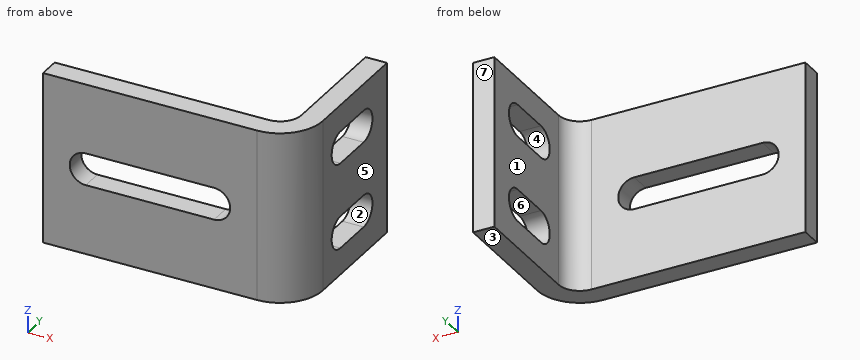
Autodesk Inventor part; units mm, degrees
ref_plane "YZ Plane" through (0, 0, 0) normal (1, 0, 0) x (0, 1, 0)
ref_plane "XZ Plane" through (0, 0, 0) normal (0, 1, 0) x (-1, 0, 0)
ref_plane "XY Plane" through (0, 0, 0) normal (0, 0, 1) x (1, 0, 0)
sketch "スケッチ1" plane through (0, 0, 0) normal (0, 1, 0) x (-1, 0, 0)
  line L0 (-10, 8) -> (10, 8)
  line L1 (10, 8) -> (10, -8)
  line L2 (10, -8) -> (-10, -8)
  line L3 (-10, -8) -> (-10, 8)
  line L4 (-10, 8) -> (10, -8) construction
  line L5 (10, 8) -> (-10, -8) construction
  point P0 (0, 0)
  dimension "d0" = 20
  dimension "d1" = 16
extrude "プレート1" add sketch "スケッチ1" along normal blind 2
sketch "スケッチ2" plane through (12, 4, -8) normal (1, 0, 0) x (0, 1, 0)
  line L0 (0, 16) -> (0, 0)
  line L1 (0, 0) -> (11, 0)
  line L2 (11, 0) -> (11, 16)
  line L3 (11, 16) -> (0, 16)
edge flange "フランジ1" height 15 angle 90 thickness 2 bend radius 2 thickness toward (1, 0, 0) relief tear relief width 2 relief depth 1 edges at (10, 2, 0) wall of the first edge with corners at (12, 4, 8) (12, 4, -8) (12, 15, -8) (12, 15, 8)
bend "曲げ1"
corner "コーナー1"
sketch "スケッチ3" plane through (14, 15, 8) normal (1, 0, 0) x (0, 0, -1)
  line L0 (2.5, -4) -> (2.5, -8)
  arc A0 (2.5, -8) -> (5.5, -8) centre (4, -8) ccw
  line L1 (5.5, -8) -> (5.5, -4)
  arc A1 (5.5, -4) -> (2.5, -4) centre (4, -4) ccw
  line L2 (10.5, -4) -> (10.5, -8)
  arc A2 (10.5, -8) -> (13.5, -8) centre (12, -8) ccw
  line L3 (13.5, -8) -> (13.5, -4)
  arc A3 (13.5, -4) -> (10.5, -4) centre (12, -4) ccw
  line L4 (0, -11) -> (0, 0)
  line L5 (16, 0) -> (16, -11)
  line L6 (0, 0) -> (16, 0)
  line L7 (0, -11) -> (16, -11)
  point P0 (8, -15)
  dimension "d13" = 4
  dimension "d14" = 4
  dimension "d17" = 3
  dimension "d18" = 4
  dimension "d19" = 1.5
  dimension "d20" = 1.5
extrude "押し出し1" cut sketch "スケッチ3" against normal blind 10 contours A1 L1 A0 L0 | A3 L3 A2 L2
sketch "スケッチ4" plane through (0, 2, 0) normal (0, 1, 0) x (1, 0, 0)
  line L0 (-6, -1.5) -> (6, -1.5)
  arc A0 (6, -1.5) -> (6, 1.5) centre (6, 0) ccw
  line L1 (6, 1.5) -> (-6, 1.5)
  arc A1 (-6, 1.5) -> (-6, -1.5) centre (-6, 0) ccw
  line L2 (-10, -8) -> (-10, 8)
  line L3 (10, 8) -> (10, -8)
  point P0 (0, 0)
  dimension "d23" = 4
  dimension "d24" = 4
  dimension "d25" = 1.5
extrude "押し出し2" cut sketch "スケッチ4" against normal blind 10
equation "\"d2\" = Thickness"
equation "\"d3\" = BendReliefWidth"
equation "\"d4\" = BendReliefDepth"
equation "\"d5\" = MinimumRemnant"
equation "\"d6\" = TransitionRadius"
equation "\"d9\" = BendRadius"
equation "\"d10\" = CornerReliefSize"
equation "\"d11\" = GapSize"
equation "\"d12\" = JacobiRadiusSize"
equation "\"BendRadius\" = Thickness"
equation "\"BendReliefWidth\" = Thickness"
equation "\"BendReliefDepth\" = 0.5 * Thickness"
equation "\"CornerReliefSize\" = 4 * Thickness"
equation "\"MinimumRemnant\" = 2 * Thickness"
equation "\"TransitionRadius\" = BendRadius"
equation "\"JacobiRadiusSize\" = BendRadius"
equation "\"GapSize\" = Thickness"
properties part number "keyL_small" material "アルミニウム 6061"
Verification items for the finished model (mm, model axes). Face numbers are marked on the shaded views. A direction names the side the tool comes from. Round coordinates to 2 decimals unless told otherwise and drop trailing zeros. Order: outer loops, then holes, each group sorted by start corner. A loop starts at its lowest first (then second) coordinate and runs counter-clockwise, first axis right, second up. Notation, with made-up numbers: (70, -15) -> (76, -15) arc R25 cw to (76, 9) -> close; hole circle Ø10 at (8, -21.5). An arc over 180 degrees is marked (long way). Put each result on its own line as item: value.
1) Depth check by flat-ended pin: pin 1 (3 mm diameter, centred on x = 3.5, z = -4, fed in from +Y); pin 2 (6 mm diameter, centred on y = 9.5, z = -5.5, fed in from -X). Enter the tip coordinate at first touch or a pass-through.
Final values:
pin 1: stops at y = 2
pin 2: stops at x = 12
2) Section check D-D (z = 6.5). Record the cut outline in (x, y).
Final values:
outline: (-10, 0) -> (10, 0) arc R4 ccw to (14, 4) -> (14, 15) -> (12, 15) -> (12, 4) arc R2 cw to (10, 2) -> (-10, 2) -> close
3) Set-up check for the marked faces 1, 2 and 3: record each of +Z, -Z, +X, -X, +Y, -Y from which the full face is reachable in a straight line by a thin tool's end or side.
Final values:
face 1: +Z, -Z, -X, +Y
face 2: +X, -X
face 3: -Z, +X, -X, +Y, -Y
4) Section check A-A (y = 8.25). Record the cut outline in (x, z).
Final values:
outline: (12, -8) -> (14, -8) -> (14, -5.5) -> (12, -5.5) -> close; (12, -2.5) -> (14, -2.5) -> (14, 2.5) -> (12, 2.5) -> close; (12, 5.5) -> (14, 5.5) -> (14, 8) -> (12, 8) -> close
5) Section check B-B (x = 2.75). Record the cut outline in (y, z), then the cut area to 3 significant figures.
Final values:
outline: (0, -8) -> (2, -8) -> (2, -1.5) -> (0, -1.5) -> close; (0, 1.5) -> (2, 1.5) -> (2, 8) -> (0, 8) -> close
area: 26.0 mm^2
6) Section check C-C (z = 0). Record the cut outline in (x, y).
Final values:
outline: (-10, 0) -> (-7.5, 0) -> (-7.5, 2) -> (-10, 2) -> close; (7.5, 0) -> (10, 0) arc R4 ccw to (14, 4) -> (14, 15) -> (12, 15) -> (12, 4) arc R2 cw to (10, 2) -> (7.5, 2) -> close
7) Mould release check, pull along Y, two halves, no side actions. Record for the marked faces 4, 5, 6 and 7: +Y half, -Y half, draft (parallel to the pull), parting line (faces both ways), or undercut.
Final values:
face 4: undercut
face 5: draft
face 6: undercut
face 7: +Y half
8) Material ranges on line 1 (Z direction, x = 12.25, y = 7.25); line 2 (Z direction, x = -6, y = 1.75); line 3 (X direction, y = 14, z = -3.75), recorded low to high.
Final values:
line 1: z = -8 to -5.5, -2.5 to 2.5, 5.5 to 8
line 2: z = -8 to -1.5, 1.5 to 8
line 3: x = 12 to 14
